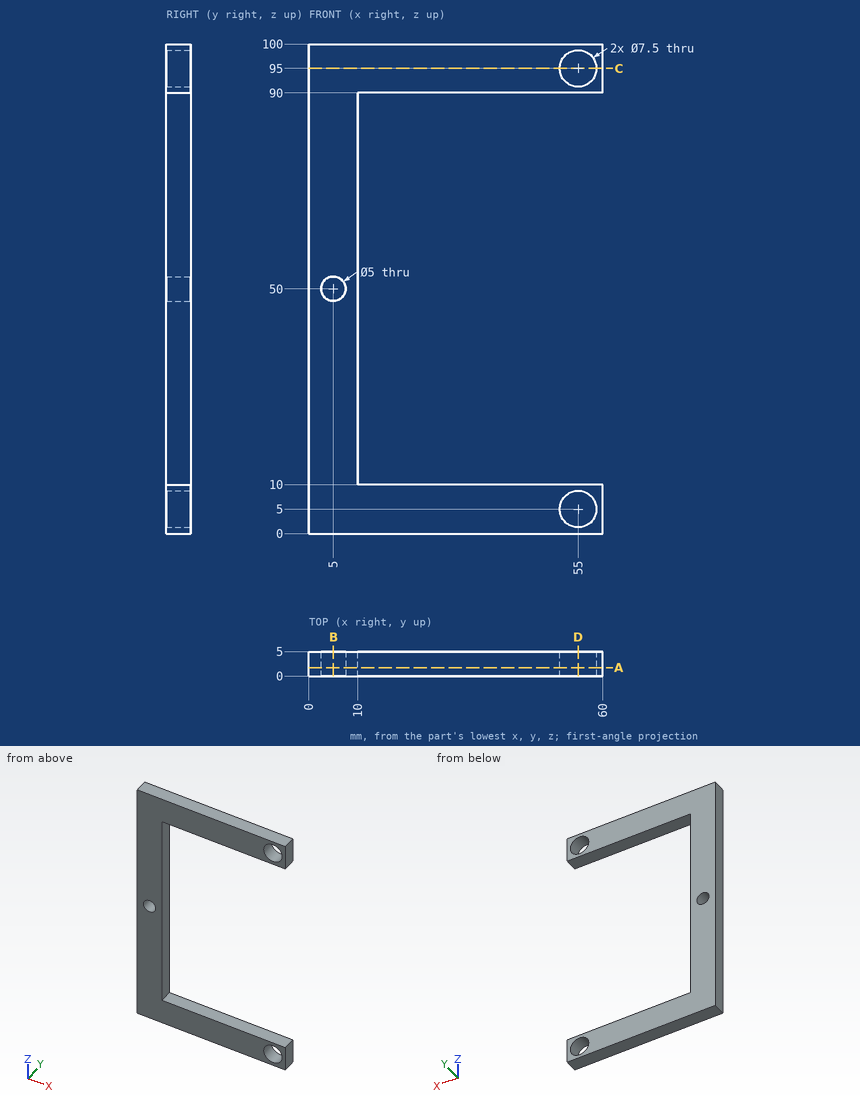
Check sheet for the drawn part. Datum: minimum x, y, z corner. Units: mm. Round coordinates to 2 decimals unless told otherwise and drop trailing zeros. Loops run counter-clockwise (first coordinate to the right, second up) from the corner with the lowest first, then second, coordinate; pieces in that order, holes last.
Item 1: Cross-section at C-C on z = 95. Record the boundary of the cut face in (x, y).
Item 2: Thickness scan on line 1 (Z direction, x = 55, y = 3.5); line 2 (X direction, y = 1.05, z = 5); line 3 (X direction, y = 2.4, z = 50). Record the ranges inside material, lowest first.
Item 3: Cross-section at D-D on x = 55. Record the boundary of the cut face in (y, z).
Item 4: Cross-section at A-A on y = 1.7. Record the boundary of the cut face in (x, z).
Item 5: Cross-section at B-B on x = 5. Record the boundary of the cut face in (y, z), then the cut area to 3 significant figures.
Answer sheet:
1. outline: (0, 0) - (51.25, 0) - (51.25, 5) - (0, 5) - close; (58.75, 0) - (60, 0) - (60, 5) - (58.75, 5) - close
2. line 1: z = 0 to 1.25, 8.75 to 10, 90 to 91.25, 98.75 to 100
2. line 2: x = 0 to 51.25, 58.75 to 60
2. line 3: x = 0 to 2.5, 7.5 to 10
3. outline: (0, 0) - (5, 0) - (5, 1.25) - (0, 1.25) - close; (0, 8.75) - (5, 8.75) - (5, 10) - (0, 10) - close; (0, 90) - (5, 90) - (5, 91.25) - (0, 91.25) - close; (0, 98.75) - (5, 98.75) - (5, 100) - (0, 100) - close
4. outline: (0, 0) - (60, 0) - (60, 10) - (10, 10) - (10, 90) - (60, 90) - (60, 100) - (0, 100) - close; hole circle Ø5 at (5, 50); hole circle Ø7.5 at (55, 5); hole circle Ø7.5 at (55, 95)
5. outline: (0, 0) - (5, 0) - (5, 47.5) - (0, 47.5) - close; (0, 52.5) - (5, 52.5) - (5, 100) - (0, 100) - close
5. area: 475 mm2
